The drawing under review shows one solid part. Ordinate dimensions are in mm from its lowest x, y, z. A direction names the side the tool comes from. Coordinates: 2 decimals unless noted, no trailing zeros. Order: outer loops, then holes, each group sorted by start corner. A loop starts at its lowest first (then second) coordinate and runs counter-clockwise, first axis right, second up.
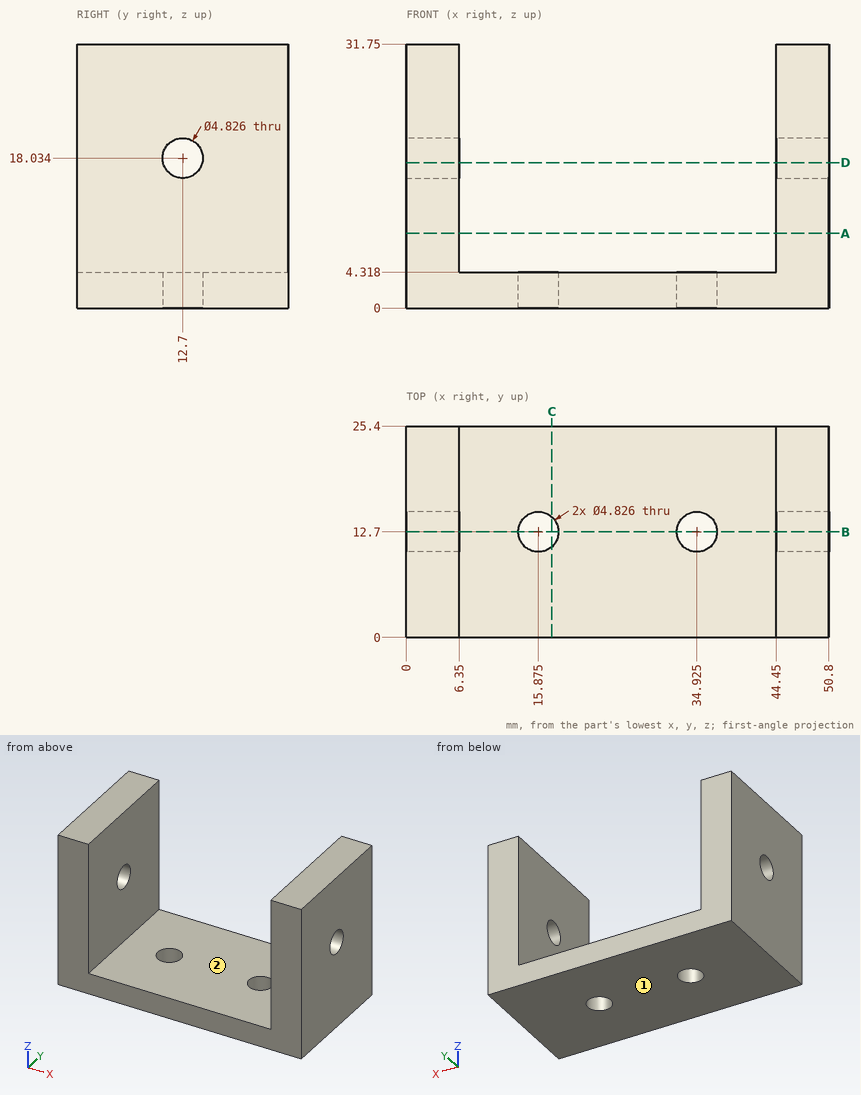
(1) Wall thickness on probe 1 along X at (y, z) = (18.75, 15); probe 2 along Z at (x, y) = (48.25, 12.7); probe 3 along Z at (x, y) = (34, 23): over which ranges is each line inside the solid? List them lowest first.
A:
probe 1: x = 0 to 6.35, 44.45 to 50.8
probe 2: z = 0 to 15.62, 20.45 to 31.75
probe 3: z = 0 to 4.32
(2) We need section D-D, the plane z = 17.5. Write out the cut boundary in (x, y), and give its area (3 significant figures).
A:
outline: (0, 0) - (6.35, 0) - (6.35, 10.35) - (0, 10.35) - close; (0, 15.05) - (6.35, 15.05) - (6.35, 25.4) - (0, 25.4) - close; (44.45, 0) - (50.8, 0) - (50.8, 10.35) - (44.45, 10.35) - close; (44.45, 15.05) - (50.8, 15.05) - (50.8, 25.4) - (44.45, 25.4) - close
area: 263 mm2
(3) Machinability: for the marked faces 1 and 2, which of the approach directions +Z, -Z, +X, -X, +Y, -Y give a long, thin tool a straight path to every point of the face, cutting with its end or side? Answer none if there is none.
A:
face 1: -Z, +X, -X, +Y, -Y
face 2: +Z, +Y, -Y
(4) We need section B-B, the plane y = 12.7. Write out the cut boundary in (x, z).
A:
outline: (0, 0) - (13.46, 0) - (13.46, 4.32) - (6.35, 4.32) - (6.35, 15.62) - (0, 15.62) - close; (0, 20.45) - (6.35, 20.45) - (6.35, 31.75) - (0, 31.75) - close; (18.29, 0) - (32.51, 0) - (32.51, 4.32) - (18.29, 4.32) - close; (37.34, 0) - (50.8, 0) - (50.8, 15.62) - (44.45, 15.62) - (44.45, 4.32) - (37.34, 4.32) - close; (44.45, 20.45) - (50.8, 20.45) - (50.8, 31.75) - (44.45, 31.75) - close
(5) We need section A-A, the plane z = 9. Write out the cut boundary in (x, y).
A:
outline: (0, 0) - (6.35, 0) - (6.35, 25.4) - (0, 25.4) - close; (44.45, 0) - (50.8, 0) - (50.8, 25.4) - (44.45, 25.4) - close
(6) For pin 1 Ø8 at (x, y) = (37.5, 12) entering from +Z, flat-tipped, find the tip position at first contact; note if it passes through.
A:
pin 1: stops at z = 4.32
(7) We need section C-C, the plane x = 17.5. Write out the cut boundary in (y, z).
A:
outline: (0, 0) - (10.92, 0) - (10.92, 4.32) - (0, 4.32) - close; (14.48, 0) - (25.4, 0) - (25.4, 4.32) - (14.48, 4.32) - close
